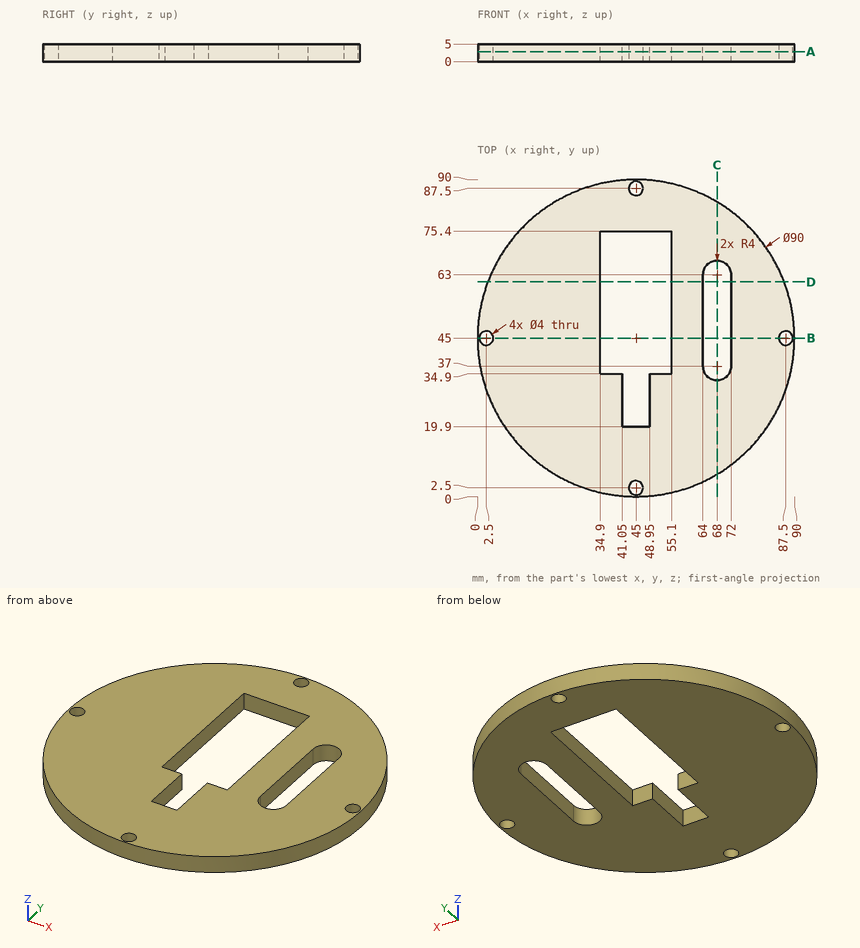
For this review, use the dimensioned drawing (mm, ordinates from the lowest corner) and the shaded views. Round coordinates to 2 decimals unless told otherwise and drop trailing zeros. Write each loop counter-clockwise with the first axis right and the second up, starting at its lowest first coordinate (ties: lowest second). Pieces come first, ordered by that corner, then holes. Notation, with made-up numbers: (-13, -11.75) -> (10, -11.75) arc R30 ccw to (10, 25.25) -> close; hole circle Ø9 at (-30, -38). An arc over 180 degrees is marked (long way). Use CSV: the item, a comma, the result in double quotes.
Q1. Consider section A-A (z = 2.85). Give the boundary of the cut face in (x, y), then the cut area to 3 significant figures.
Checks:
outline,"circle Ø90 at (45, 45); hole circle Ø4 at (2.5, 45); hole (34.9, 34.9) -> (41.05, 34.9) -> (41.05, 19.9) -> (48.95, 19.9) -> (48.95, 34.9) -> (55.1, 34.9) -> (55.1, 75.4) -> (34.9, 75.4) -> close; hole circle Ø4 at (45, 2.5); hole circle Ø4 at (45, 87.5); hole (64, 37) arc R4 ccw to (72, 37) -> (72, 63) arc R4 ccw to (64, 63) -> close; hole circle Ø4 at (87.5, 45)"
area,"5,120 mm²"
Q2. Consider section C-C (x = 68). Give the boundary of the cut face in (y, z).
Checks:
outline,"(6.32, 0) -> (33, 0) -> (33, 5) -> (6.32, 5) -> close; (67, 0) -> (83.68, 0) -> (83.68, 5) -> (67, 5) -> close"
Q3. For pin 1 Ø2 at (x, z) = (78.5, 4) entering from -Y; pin 2 Ø3 at (x, y) = (45, 87.5) entering from +Z; pin 3 Ø2.5 at (y, z) = (55.5, 2.5) entering from -X; pin 4 Ø2.5 at (y, z) = (31, 2.5) entering from -X, all flat-tipped, find the tip position at first contact; note any pin that passes through.
Checks:
pin 1,"y = 13.88"
pin 2,"through"
pin 3,"x = 0.96"
pin 4,"x = 1.84"
Q4. Consider section B-B (y = 45). Give the boundary of the cut face in (x, z).
Checks:
outline,"(0, 0) -> (0.5, 0) -> (0.5, 5) -> (0, 5) -> close; (4.5, 0) -> (34.9, 0) -> (34.9, 5) -> (4.5, 5) -> close; (55.1, 0) -> (64, 0) -> (64, 5) -> (55.1, 5) -> close; (72, 0) -> (85.5, 0) -> (85.5, 5) -> (72, 5) -> close; (89.5, 0) -> (90, 0) -> (90, 5) -> (89.5, 5) -> close"
Q5. Consider section D-D (y = 61). Give the boundary of the cut face in (x, z).
Checks:
outline,"(2.94, 0) -> (34.9, 0) -> (34.9, 5) -> (2.94, 5) -> close; (55.1, 0) -> (64, 0) -> (64, 5) -> (55.1, 5) -> close; (72, 0) -> (87.06, 0) -> (87.06, 5) -> (72, 5) -> close"
Q6. To check wall thickness, follow probe 1 along Y at (x, z) = (45, 1.8); probe 2 along Y at (x, z) = (44.5, 4); probe 3 along X at (y, z) = (59, 4.45). State the ranges of each line that lie inside material, in increasing order. Write a range as [from, to].
Checks:
probe 1,"[0, 0.5], [4.5, 19.9], [75.4, 85.5], [89.5, 90]"
probe 2,"[0, 0.56], [4.44, 19.9], [75.4, 85.56], [89.44, 90]"
probe 3,"[2.23, 34.9], [55.1, 64], [72, 87.77]"
